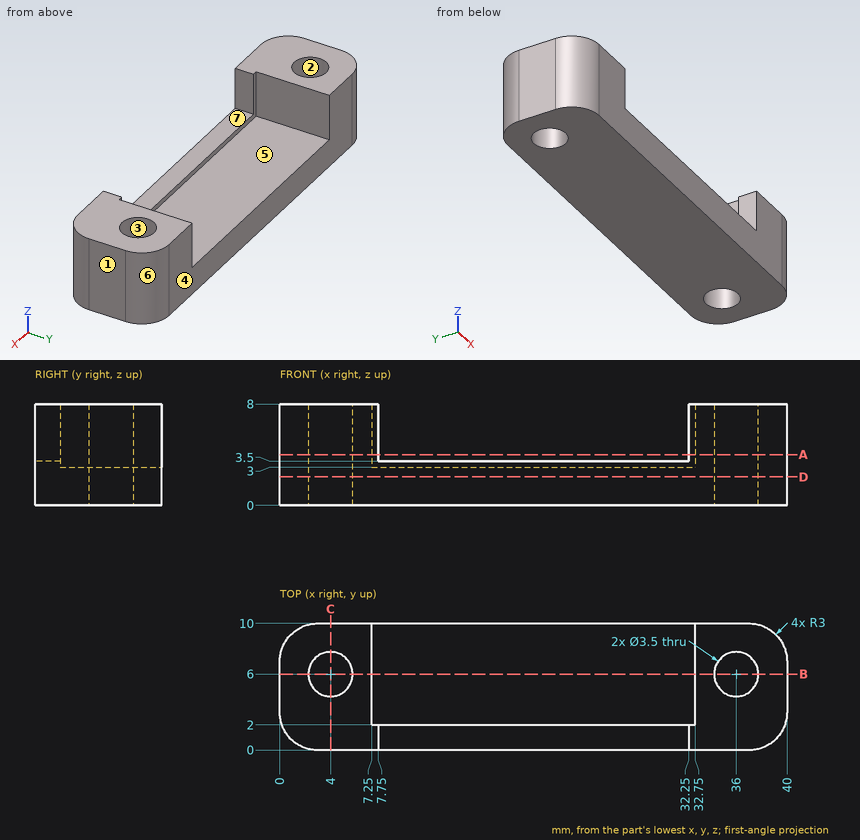
Could you check a few things on this drawing? It's one solid part, dimensions in mm from its lowest x, y, z. A direction names the side the tool comes from. Coordinates: 2 decimals unless noted, no trailing zeros. Write each loop counter-clockwise with the first axis right and the second up, starting at its lowest first coordinate (ties: lowest second). Pieces come first, ordered by that corner, then holes.
Q1. Imagine slicing it at D-D, the plane z = 2.25. List the corners of the cut face in (x, y) for me, plus the area to 3 significant figures.
Results found:
outline: (0, 3) arc R3 ccw to (3, 0) - (37, 0) arc R3 ccw to (40, 3) - (40, 7) arc R3 ccw to (37, 10) - (3, 10) arc R3 ccw to (0, 7) - close; hole circle Ø3.5 at (4, 6); hole circle Ø3.5 at (36, 6)
area: 373 mm2
Q2. Imagine slicing it at C-C, the plane x = 4. List the corners of the cut face in (y, z) for me.
Results found:
outline: (0, 0) - (4.25, 0) - (4.25, 8) - (0, 8) - close; (7.75, 0) - (10, 0) - (10, 8) - (7.75, 8) - close
Q3. Please list where these lines run through material, in increasing order: L1, parallel to Y at x = 4, z = 5.25; L2, parallel to X at y = 7.5, z = 7.5; L3, parallel to Z at x = 12, y = 4.5.
Results found:
L1: y = 0 to 4.25, 7.75 to 10
L2: x = 0.04 to 3.1, 4.9 to 7.25, 32.75 to 35.1, 36.9 to 39.96
L3: z = 0 to 3
Q4. Imagine slicing it at A-A, the plane z = 4. List the corners of the cut face in (x, y) for me, plus the area to 3 significant figures.
Results found:
outline: (0, 3) arc R3 ccw to (3, 0) - (7.75, 0) - (7.75, 2) - (7.25, 2) - (7.25, 10) - (3, 10) arc R3 ccw to (0, 7) - close; (32.25, 0) - (37, 0) arc R3 ccw to (40, 3) - (40, 7) arc R3 ccw to (37, 10) - (32.75, 10) - (32.75, 2) - (32.25, 2) - close; hole circle Ø3.5 at (4, 6); hole circle Ø3.5 at (36, 6)
area: 120 mm2
Q5. Which directions (+Z, -Z, +X, -X, +Y, -Y) give clear straight access to the entire face, cutting with the end or side of a thin tool? Please do the marked faces 5, 6 and 7.
Results found:
face 5: +Z, +Y
face 6: +Z, -Z, +X, +Y
face 7: +Z, +Y, -Y
Q6. For P1, Ø5, axis at x = 14, y = 6.5, coming from the +Z side; P2, Ø0.6, axis at y = 0.5, z = 6.5, coming from the -X side; P3, Ø3, axis at x = 4, y = 6, coming from the +Z side; P4, Ø0.6, axis at y = 1, z = 6, coming from the +X side, each with a flat end and sliding along its axis, tell me the tip position at first contact or that it passes through.
Results found:
P1: stops at z = 3
P2: stops at x = 0.96
P3: passes through
P4: stops at x = 39.47
Q7. Imagine slicing it at B-B, the plane y = 6. List the corners of the cut face in (x, z) for me.
Results found:
outline: (0, 0) - (2.25, 0) - (2.25, 8) - (0, 8) - close; (5.75, 0) - (34.25, 0) - (34.25, 8) - (32.75, 8) - (32.75, 3) - (7.25, 3) - (7.25, 8) - (5.75, 8) - close; (37.75, 0) - (40, 0) - (40, 8) - (37.75, 8) - close
Q8. If we mould it in two halves opening along Y, with no side actions, what happens to the marked faces 1, 2, 3 and 4? For each: +Y half, -Y half, draft (parallel to the pull), parting line (faces both ways), or undercut.
Results found:
face 1: draft
face 2: undercut
face 3: undercut
face 4: +Y half
